from build123d import *

# Parameters (mm, degrees)
F1_DEPTH         = 38.1
F3_DEPTH         = 12.7
F3_COPIES1_COUNT = 2
F5_DEPTH         = 101.601
F7_D             = 11.5062
F7_DEPTH         = 38.1
F7_TIP           = 3.4568112273
F9_DEPTH         = 101.601


# Not quite as in the source:
# - a pattern or mirror of a feature is missing from the dataset's text; its kind, count and spacing are read off the source's solid


with BuildPart() as f1:
    # F0 (on Front) → F1 (new body, symmetric)
    with BuildSketch(Plane.XZ):
        Polygon((-114.3, 38.1), (-114.3, 0), (114.3, 0), (114.3, 38.1), (88.9, 38.1), (88.9, 63.5), (-88.9, 63.5), (-88.9, 38.1), align=None)
    extrude(amount=F1_DEPTH, both=True)

    # F2 (on face) → F3 (join)
    with BuildSketch(Plane.XZ.offset(38.1)):
        with BuildLine():
            Line((19.05, 31.75), (44.45, 31.75))
            ThreePointArc((44.45, 31.75), (66.9006403027, 41.0493596973), (76.2, 63.5))
            Line((76.2, 63.5), (0, 63.5))
            Line((0, 63.5), (0, 0))
            Line((0, 0), (19.05, 0))
            Line((19.05, 0), (19.05, 31.75))
        make_face()
    f3 = extrude(amount=F3_DEPTH)

    # F3_copies: F3 across plane
    add(f3.mirror(Plane(origin=(0, 0, 0), x_dir=(0, 0, -1), z_dir=(-1, 0, 0))))

    # F3_copies1: F3 ×2 about axis
    f3_copies1_axis = Axis((0, 0, 0), (0, 0, 1))
    for i in range(1, F3_COPIES1_COUNT):
        add(f3.rotate(f3_copies1_axis, i * 360 / F3_COPIES1_COUNT))

    # F3_copies2: F3 across plane
    add(f3.mirror(Plane.ZX))

    # F4 (on face) → F5 (cut, through all)
    with BuildSketch(Plane.XZ.offset(50.8)):
        Polygon((-63.5, 12.7), (-50.8, 0), (50.8, 0), (63.5, 12.7), align=None)
    extrude(amount=-F5_DEPTH, mode=Mode.SUBTRACT)

    # F7
    with Locations(Plane.XY.offset(63.5)):
        with Locations((-76.2, 19.05), (-76.2, -19.05), (0, 38.1), (0, -38.1), (76.2, -19.05), (76.2, 19.05)):
            Hole(F7_D / 2, depth=F7_DEPTH)
            with Locations((0, 0, -(F7_DEPTH + F7_TIP / 2))):  # 118° drill point
                Cone(0, F7_D / 2, F7_TIP, mode=Mode.SUBTRACT)

    # F8 (on face) → F9 (cut, through all)
    with BuildSketch(Plane.XZ.offset(50.8)):
        with BuildLine():
            Line((-25.4, 63.5), (-63.5, 63.5))
            ThreePointArc((-63.5, 63.5), (-44.45, 44.45), (-25.4, 63.5))
        make_face()
        with BuildLine():
            Line((63.5, 63.5), (25.4, 63.5))
            ThreePointArc((25.4, 63.5), (44.45, 44.45), (63.5, 63.5))
        make_face()
    extrude(amount=-F9_DEPTH, mode=Mode.SUBTRACT)


solid = f1.part
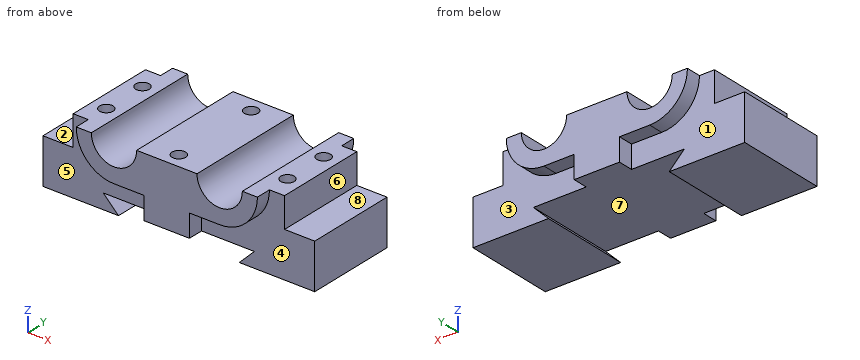
Can you work these out from the model? Positions are in its coordinate system, mm. Face numbers are marked on the shaded views. A direction names the side the tool comes from. Give positions to 0.01 mm unless a question says otherwise; leave off trailing zeros. Loops run counter-clockwise (first coordinate to the right, second up) from the corner with the lowest first, then second, coordinate; pieces in that order, holes last. Notation, with made-up numbers: M 80,-3 L 120,-3 A9 ccw 120,12 Z; hole C 19,48 d6. An arc over 180 degrees is marked long. One line per item, written item: value.
1) I'm going to push flat-ended pins straight in: pin 1 (1 mm diameter, centred on x = -32, y = 2.5, fed in from -Z); pin 2 (4 mm diameter, centred on x = 25.5, y = 47, fed in from -Z); pin 3 (8 mm diameter, centred on x = 26.5, z = 11, fed in from +Y). Where does each tip first touch, or does it pass through?
Geometry check:
pin 1: stops at z = 12.7
pin 2: stops at z = 31.75
pin 3: stops at y = 38.1
2) On a 3-axis mill with a long thin cutter (end or side, diameter ignored), from which of +Z, -Z, +X, -X, +Y, -Y can I reach the whole of each face in a straight line? I mean the marked faces 1, 2, 3, 4 and 5. Say none if no direction works.
Geometry check:
face 1: -Z, -X, +Y
face 2: +Z, -X, +Y, -Y
face 3: -Z, +X, +Y
face 4: -Z, +X, -Y
face 5: -Z, -X, -Y
3) Imagine slicing it at D-D on x = 47.5. Write out the boundary of the cut face in (y, z), and give its area (3 significant figures).
Geometry check:
outline: M -50.8,31.9 L -38.1,31.9 L -38.1,12.7 L 38.1,12.7 L 38.1,31.9 L 50.8,31.9 L 50.8,44.7 L -50.8,44.7 Z
area: 2,760 mm²
4) Imagine slicing it at C-C on y = -7. Write out the boundary of the cut face in (x, z).
Geometry check:
outline: M -114.3,0 L -50.8,0 L -63.5,12.7 L 63.5,12.7 L 50.8,0 L 114.3,0 L 114.3,38.1 L 88.9,38.1 L 88.9,63.5 L 63.5,63.5 A19.05 cw 25.4,63.5 L -25.4,63.5 A19.05 cw -63.5,63.5 L -88.9,63.5 L -88.9,38.1 L -114.3,38.1 Z
5) Imagine slicing it at B-B on x = -56. Write out the boundary of the cut face in (y, z), and give its area (3 significant figures).
Geometry check:
outline: M -50.8,33.93 L -38.1,33.93 L -38.1,12.7 L 38.1,12.7 L 38.1,33.93 L 50.8,33.93 L 50.8,48.35 L -50.8,48.35 Z; M -38.1,0 L 38.1,0 L 38.1,5.2 L -38.1,5.2 Z
area: 3,480 mm²
6) Please list where these lines run through material, in increasing order: line 1 (X direction, y = -19, z = 42); line 2 (Y direction, x = -76, z = 54); line 3 (X direction, y = 3.5, z = 57).
Geometry check:
line 1: x = -88.9 to -81.95, -70.45 to 70.45, 81.95 to 88.9
line 2: y = -38.1 to -24.8, -13.3 to 13.3, 24.8 to 38.1
line 3: x = -88.9 to -62.36, -26.54 to 26.54, 62.36 to 88.9
7) Imagine slicing it at A-A on z = 58. Count the separate pieces of the cut face and the enclosed holes in it, and give its area (3 significant figures).
Geometry check:
separate pieces: 3
enclosed holes: 6
area: 9,360 mm²
8) Thinking about a two-plate mould opening in X: for the marked faces 6, 7 and 8, which applies, +X half, -X half, draft (parallel to the pull), parting line (faces both ways), or undercut?
Geometry check:
face 6: +X half
face 7: undercut
face 8: draft
